Could you check a few things on this drawing? It's one solid part, dimensions in mm from its lowest x, y, z. Round coordinates to 2 decimals unless told otherwise and drop trailing zeros. Order: outer loops, then holes, each group sorted by start corner. A loop starts at its lowest first (then second) coordinate and runs counter-clockwise, first axis right, second up. Notation, with made-up numbers: (20.25, 67) -> (52.25, 67) arc R13 cw to (52.25, 83) -> close; hole circle Ø2 at (-30, -3.5). An arc over 180 degrees is marked (long way). Use a Markdown table: item, result. Add a question column.
(1) I'm going to push flat-ended pins straight in: P1, Ø6, axis at x = 8.5, z = 42.5, coming from the +Y side; P2, Ø1.5, axis at y = 3, z = 47, coming from the +X side; P3, Ø1.5, axis at x = 5.5, z = 17, coming from the +Y side. Where does each tip first touch, or does it pass through?
(2) I want a section at B-B, the plane y = 12.75. Please give me the cut outline in (x, z) (1 decimal).
(3) I want a section at C-C, the plane z = 20. Please give me the cut outline in (x, y), then the cut area to 3 significant figures.
(4) I want a section at A-A, the plane x = 3. Please give me the cut outline in (y, z) (1 decimal).
(5) Thinking about a two-plate mould opening in Z: for the marked faces 1, 2 and 3, which applies, pulls with the +Z half, pulls with the -Z half, needs draft (parallel to the pull), parting line crosses it, or undercut?
(6) I want a section at D-D, the plane y = 4. Please give me the cut outline in (x, z) (1 decimal), then the cut area to 3 significant figures.
(7) If I drill on probe 1 along Z at (x, y) = (4, 10.75) (1 decimal); probe 2 along X at (y, z) = (14, 30); probe 3 along Y at (x, z) = (11.75, 91.5) (1 decimal), over which ranges is the centre line in solid material (lowest first)?
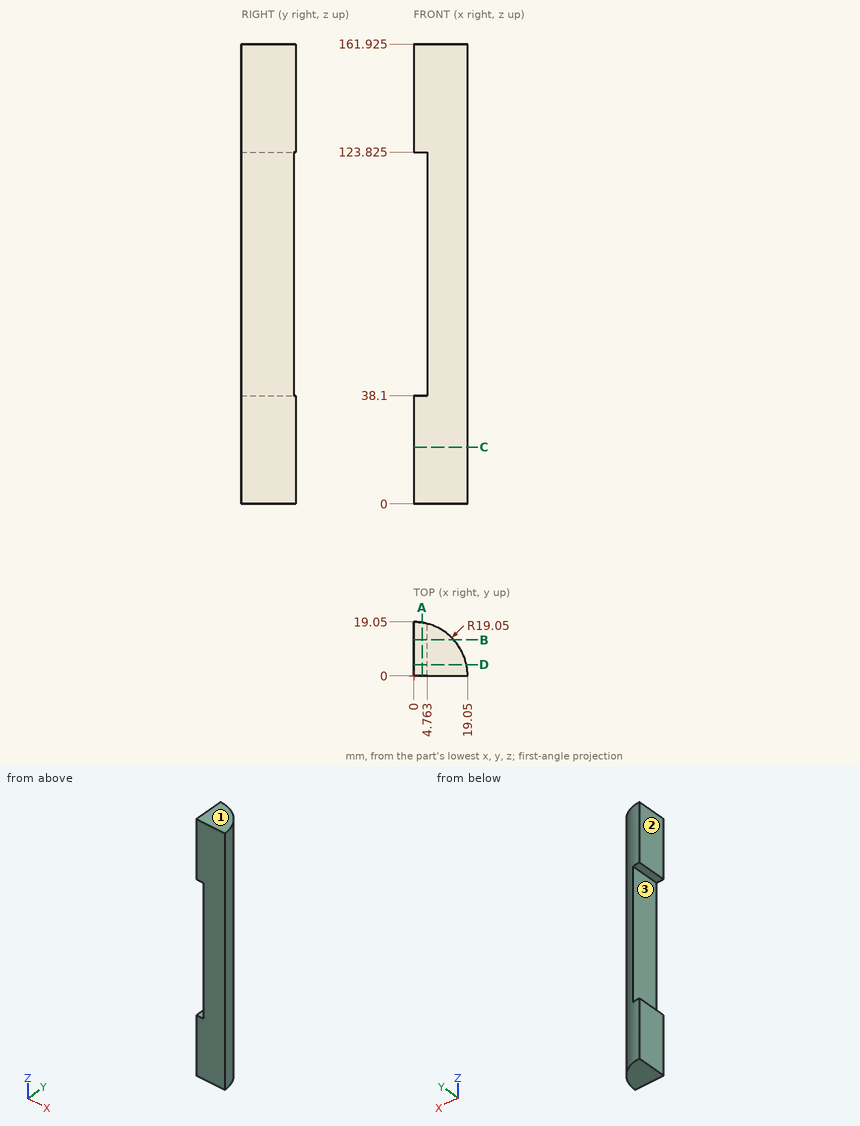
Taken from the geometry:
| question | item | result |
|---|---|---|
| 1 | P1 | stops at y = 18.24 |
| 1 | P2 | stops at x = 18.92 |
| 1 | P3 | stops at y = 18.45 |
| 2 | outline | (0, 0) -> (14.2, 0) -> (14.2, 161.9) -> (0, 161.9) -> (0, 123.8) -> (4.8, 123.8) -> (4.8, 38.1) -> (0, 38.1) -> close |
| 3 | outline | (0, 0) -> (19.05, 0) arc R19.05 ccw to (0, 19.05) -> close |
| 3 | area | 285 mm2 |
| 4 | outline | (0, 0) -> (18.8, 0) -> (18.8, 38.1) -> (0, 38.1) -> close; (0, 123.8) -> (18.8, 123.8) -> (18.8, 161.9) -> (0, 161.9) -> close |
| 5 | face 1 | pulls with the +Z half |
| 5 | face 2 | needs draft |
| 5 | face 3 | undercut |
| 6 | outline | (0, 0) -> (18.6, 0) -> (18.6, 161.9) -> (0, 161.9) -> (0, 123.8) -> (4.8, 123.8) -> (4.8, 38.1) -> (0, 38.1) -> close |
| 6 | area | 2,610 mm2 |
| 7 | probe 1 | z = 0 to 38.1, 123.8 to 161.9 |
| 7 | probe 2 | x = 0 to 12.92 |
| 7 | probe 3 | y = 0 to 15 |
